Could you check a few things on this model? Use its own coordinates, in mm. A direction names the side the tool comes from. Round coordinates to 2 decimals unless told otherwise and drop trailing zeros. Loops run counter-clockwise (first coordinate to the right, second up) from the corner with the lowest first, then second, coordinate; pieces in that order, holes last. Notation, with made-up numbers: (86, -2) - (126, -2) arc R18 ccw to (126, 11) - close; hole circle Ø3 at (61.5, -25). An arc over 180 degrees is marked (long way). Answer as CSV lines item,"result". Start each with the question number.
1) Suppose I cut it at B-B, the plane y = 2.25. Count the separate pieces of the cut face and the enclosed holes in it, then the cut area to 3 significant figures.
2) We'd pull the mould along Z, two halves only. Please class faces 1 (the face through (41.99, 1.52, -47.15)), 2 (the face through (16, 1, 15)), 3 (the face through (-45, 1, 1)): pulls with the +Z half, pulls with the -Z half, needs draft (parallel to the pull), parting line crosses it, or undercut.
3) Which directions (+Z, -Z, +X, -X, +Y, -Y) give clear straight access to the entire face, cutting with the end or side of a thin tool? Please do faces 4 (the face through (-15, 1, -40)), 5 (the face through (0, 1, -50)).
4) Suppose I cut it at C-C, the plane x = 32.3. Write out the boundary of the cut face in (y, z).
5) Suppose I cut it at A-A, the plane x = -32.3. Write out the boundary of the cut face in (y, z).
6) I'm going to push flat-ended pins straight in: pin 1 Ø1.5 at (y, z) = (1, 41) entering from +X; pin 2 Ø1.5 at (x, y) = (-40.5, 1.5) entering from +Z. Where does each tip first touch, or does it pass through?
7) Please list where these lines run through material, in increasing order: line 1 along X through (y, z) = (1.9, -19.5); line 2 along Z through (x, y) = (-32.3, 2.3); line 3 along Z through (x, y) = (31.5, 2.5).
```python
from build123d import *

# Parameters (mm, degrees)
SKETCH2_W           = 90
SKETCH2_H           = 100
SKETCH2_R           = 3.5685
SKETCH2_R_2         = 2.75
SKETCH2_W_2         = 3
SKETCH2_H_2         = 5
SKETCH2_H_3         = 10
BOSS_EXTRUDE1_DEPTH = 3
FILLET1_R           = 10


with BuildPart() as part:
    # Sketch2 → Boss-Extrude1 (new body)
    with BuildSketch(Plane(origin=(0, 0, 0), x_dir=(1, 0, 0), z_dir=(0, 1, 0))):
        Rectangle(SKETCH2_W, SKETCH2_H)
        with Locations((-32.3, 40)):
            Circle(SKETCH2_R, mode=Mode.SUBTRACT)
        with Locations((-32.3, -40)):
            Circle(SKETCH2_R, mode=Mode.SUBTRACT)
        with Locations((32.3, 40)):
            Circle(SKETCH2_R_2, mode=Mode.SUBTRACT)
        with Locations((32.3, -40)):
            Circle(SKETCH2_R_2, mode=Mode.SUBTRACT)
        with Locations((39.8, 40)):
            Rectangle(SKETCH2_W_2, SKETCH2_H_2, mode=Mode.SUBTRACT)
        with Locations((-16.5, 20)):
            Rectangle(SKETCH2_W_2, SKETCH2_H_3, mode=Mode.SUBTRACT)
        with Locations((-16.5, 0)):
            Rectangle(SKETCH2_W_2, SKETCH2_H_3, mode=Mode.SUBTRACT)
        with Locations((-16.5, 40)):
            Rectangle(SKETCH2_W_2, SKETCH2_H_3, mode=Mode.SUBTRACT)
        with Locations((-16.5, -20)):
            Rectangle(SKETCH2_W_2, SKETCH2_H_3, mode=Mode.SUBTRACT)
        with Locations((-16.5, -40)):
            Rectangle(SKETCH2_W_2, SKETCH2_H_3, mode=Mode.SUBTRACT)
        with Locations((16.5, -40)):
            Rectangle(SKETCH2_W_2, SKETCH2_H_3, mode=Mode.SUBTRACT)
        with Locations((16.5, -20)):
            Rectangle(SKETCH2_W_2, SKETCH2_H_3, mode=Mode.SUBTRACT)
        with Locations((16.5, 40)):
            Rectangle(SKETCH2_W_2, SKETCH2_H_3, mode=Mode.SUBTRACT)
        with Locations((16.5, 20)):
            Rectangle(SKETCH2_W_2, SKETCH2_H_3, mode=Mode.SUBTRACT)
        with Locations((16.5, 0)):
            Rectangle(SKETCH2_W_2, SKETCH2_H_3, mode=Mode.SUBTRACT)
        with Locations((-39.8, 40)):
            Rectangle(SKETCH2_W_2, SKETCH2_H_2, mode=Mode.SUBTRACT)
        with Locations((39.8, -40)):
            Rectangle(SKETCH2_W_2, SKETCH2_H_2, mode=Mode.SUBTRACT)
        with Locations((-39.8, -40)):
            Rectangle(SKETCH2_W_2, SKETCH2_H_2, mode=Mode.SUBTRACT)
        with Locations((-24.8, -40)):
            Rectangle(SKETCH2_W_2, SKETCH2_H_2, mode=Mode.SUBTRACT)
        with Locations((-24.8, 40)):
            Rectangle(SKETCH2_W_2, SKETCH2_H_2, mode=Mode.SUBTRACT)
        with Locations((24.8, 40)):
            Rectangle(SKETCH2_W_2, SKETCH2_H_2, mode=Mode.SUBTRACT)
        with Locations((24.8, -40)):
            Rectangle(SKETCH2_W_2, SKETCH2_H_2, mode=Mode.SUBTRACT)
    extrude(amount=BOSS_EXTRUDE1_DEPTH)

    # Fillet1
    fillet1_edges = [part.edges().sort_by_distance(p)[0] for p in [
        (-45, 1.5, -50),
        (45, 1.5, -50),
        (45, 1.5, 50),
        (-45, 1.5, 50),
    ]]
    fillet(fillet1_edges, radius=FILLET1_R)


solid = part.part
```
Filled sheet:
1,separate pieces,"1"
1,enclosed holes,"22"
1,area,"8,370 mm²"
2,face 1,"pulls with the -Z half"
2,face 2,"undercut"
2,face 3,"needs draft"
3,face 4,"+Y, -Y"
3,face 5,"-Z, +X, -X, +Y, -Y"
4,outline,"(0, -50) - (3, -50) - (3, -42.75) - (0, -42.75) - close; (0, -37.25) - (3, -37.25) - (3, 37.25) - (0, 37.25) - close; (0, 42.75) - (3, 42.75) - (3, 50) - (0, 50) - close"
5,outline,"(0, -50) - (3, -50) - (3, -43.57) - (0, -43.57) - close; (0, -36.43) - (3, -36.43) - (3, 36.43) - (0, 36.43) - close; (0, 43.57) - (3, 43.57) - (3, 50) - (0, 50) - close"
6,pin 1,"x = 45"
6,pin 2,"z = 48.8"
7,line 1,"-45 to -18, -15 to 15, 18 to 45"
7,line 2,"-50 to -43.57, -36.43 to 36.43, 43.57 to 50"
7,line 3,"-50 to -42.63, -37.37 to 37.37, 42.63 to 50"
